```python
from build123d import *

# Parameters (mm, degrees)
SKETCH_1_W          = 60
SKETCH_1_H          = 25
EXTRUDE_1_DEPTH     = 1
SKETCH_2_R          = 1.5
CUT_EXTRUDE_1_DEPTH = 2
FILLET_1_R          = 2


with BuildPart() as part:
    # ｽｹｯﾁ1 → ﾎﾞｽ - 押し出し1 (new body)
    with BuildSketch(Plane.XY):
        Rectangle(SKETCH_1_W, SKETCH_1_H)
    extrude(amount=EXTRUDE_1_DEPTH)

    # ｽｹｯﾁ2 → ｶｯﾄ - 押し出し1 (cut, through all)
    with BuildSketch(Plane.XY.offset(1)):
        with Locations((-27, 9.5)):
            Circle(SKETCH_2_R)
        with Locations((27, 9.5)):
            Circle(SKETCH_2_R)
        with Locations((-27, -9.5)):
            Circle(SKETCH_2_R)
        with Locations((27, -9.5)):
            Circle(SKETCH_2_R)
    extrude(amount=-CUT_EXTRUDE_1_DEPTH, mode=Mode.SUBTRACT)

    # ﾌｨﾚｯﾄ1
    fillet_1_edges = [part.edges().sort_by_distance(p)[0] for p in [
        (-30, 12.5, 0.5),
        (30, 12.5, 0.5),
        (30, -12.5, 0.5),
        (-30, -12.5, 0.5),
    ]]
    fillet(fillet_1_edges, radius=FILLET_1_R)


solid = part.part
```
CAD build for the part. Positions are in the model's coordinates, mm. Round coordinates to 2 decimals unless told otherwise and drop trailing zeros. Order: outer loops, then holes, each group sorted by start corner. A loop starts at its lowest first (then second) coordinate and runs counter-clockwise, first axis right, second up.
Q1. Wall check: L1, parallel to Y at x = 27, z = 0.7; L2, parallel to X at y = 10.5, z = 0.85; L3, parallel to Y at x = -26, z = 0.9. Give the ranges that are in metal, low to high.
Q2. Slice it at B-B (x = -27). Write the cut outline in (y, z).
Q3. Slice it at A-A (y = -9.5). Write the cut outline in (x, z), and give its area (3 significant figures).
Q4. Slice it at C-C (z = 0.55). Write the cut outline in (x, y), and give its area (3 significant figures).
Q5. Two-plate mould, pull along X, no slides. Class faces 1 (the flat face through (0, 0, 0)), 2 (the cylindrical face through (-29.43, -11.9, 0.51)), 3 (the cylindrical face through (25.5, -9.43, 0.51)): pulls with the +X half, pulls with the -X half, needs draft (parallel to the pull), parting line crosses it, or undercut.
Results below:
1. L1: y = -12.5 to -11, -8 to 8, 11 to 12.5
1. L2: x = -30 to -28.12, -25.88 to 25.88, 28.12 to 30
1. L3: y = -12.5 to -10.62, -8.38 to 8.38, 10.62 to 12.5
2. outline: (-12.5, 0) - (-11, 0) - (-11, 1) - (-12.5, 1) - close; (-8, 0) - (8, 0) - (8, 1) - (-8, 1) - close; (11, 0) - (12.5, 0) - (12.5, 1) - (11, 1) - close
3. outline: (-30, 0) - (-28.5, 0) - (-28.5, 1) - (-30, 1) - close; (-25.5, 0) - (25.5, 0) - (25.5, 1) - (-25.5, 1) - close; (28.5, 0) - (30, 0) - (30, 1) - (28.5, 1) - close
3. area: 54.0 mm2
4. outline: (-30, -10.5) arc R2 ccw to (-28, -12.5) - (28, -12.5) arc R2 ccw to (30, -10.5) - (30, 10.5) arc R2 ccw to (28, 12.5) - (-28, 12.5) arc R2 ccw to (-30, 10.5) - close; hole circle Ø3 at (-27, -9.5); hole circle Ø3 at (-27, 9.5); hole circle Ø3 at (27, -9.5); hole circle Ø3 at (27, 9.5)
4. area: 1,470 mm2
5. face 1: needs draft
5. face 2: pulls with the -X half
5. face 3: undercut
